Work out the finished part from the listing and answer in its coordinate system (mm). A direction names the side the tool comes from. Coordinates: 2 decimals unless noted, no trailing zeros. Loops run counter-clockwise (first coordinate to the right, second up) from the corner with the lowest first, then second, coordinate; pieces in that order, holes last. Notation, with made-up numbers: (-19, -35.75) -> (11, -35.75) arc R19 ccw to (11, -12.75) -> close; hole circle Ø1 at (1.5, 12). An arc over 180 degrees is marked (long way). One line per question, with ' | ' between items.
```python
from build123d import *

# Parameters (mm, degrees)
F3_R = 12


with BuildPart() as f1:
    # F0 (on Front) → F1 (revolve)
    with BuildSketch(Plane.XZ):
        Polygon((-12, 0), (-10, 0), (-10, 50), (0, 50), (0, 60), (-12, 60), align=None)
    revolve(axis=Axis((0, 0, 25), (0, 0, -1)))

    # F4: sweep along a path in F2
    with BuildLine(Plane.XZ) as f4_path:
        Line((0, 60), (-31.715729, 60))
        ThreePointArc((-31.715729, 60), (-39.369397, 61.522409), (-45.857864, 65.857864))
        Line((-45.857864, 65.857864), (-65.857864, 85.857864))
        ThreePointArc((-65.857864, 85.857864), (-70.193319, 107.653669), (-51.715729, 120))
        Line((-51.715729, 120), (51.715729, 120))
        ThreePointArc((51.715729, 120), (70.193319, 107.653669), (65.857864, 85.857864))
        Line((65.857864, 85.857864), (45.857864, 65.857864))
        ThreePointArc((45.857864, 65.857864), (39.369397, 61.522409), (31.715729, 60))
        Line((31.715729, 60), (0, 60))
    # F3 (on Right) → F4 (sweep)
    with BuildSketch(Plane.YZ):
        with Locations((0, 60)):
            Circle(F3_R)
    sweep(path=f4_path.line)


solid = f1.part
```
1) Flat-ended cylindrical pins translate along their axes: pin 1 (1 mm diameter, centred on x = -33, y = 5.5, fed in from +Z); pin 2 (4 mm diameter, centred on y = 4, z = 55.5, fed in from -X); pin 3 (12 mm diameter, centred on x = 29, z = 73, fed in from +Y). Find the tip coordinate at first contact, or state that the pin passes through.
Check values:
pin 1: stops at z = 130.91 | pin 2: stops at x = -53.69 | pin 3: stops at y = 9.75
2) Find the intervals of material crossed by line 1 along Y through (x, z) = (0, 36); line 2 along Z through (x, y) = (-47, -3.5); line 3 along Z through (x, y) = (36, 10), in increasing order.
Check values:
line 1: y = -12 to -10, 10 to 12 | line 2: z = 52.48 to 83.23, 108.52 to 131.48 | line 3: z = 53.71 to 67.34, 113.37 to 126.63
3) Find section A-A (z = 22). Write down the section's boundary in (x, y), plus the area to 3 significant figures.
Check values:
outline: circle Ø24 at (0, 0); hole circle Ø20 at (0, 0) | area: 138 mm^2
4) The mould has two halves that part along X. Classify faces 3 (the face through (0, -8, 50)), 4 (the face through (11.99, 0.53, 22.91)), 5 (the face through (5, 9, 0)): released by +X, released by -X, zero draft, split by the parting line, or undercut.
Check values:
face 3: undercut | face 4: split by the parting line | face 5: zero draft
5) For faces 1 (the face through (-0.444, 5.537, 70.646)), 2 (the face through (0, 8, 50)), determine the directions among +Z, -Z, +X, -X, +Y, -Y from which every point of the face is accessible in a straight line to the end or side of a thin tool.
Check values:
face 1: none | face 2: -Z
